```python
from build123d import *

# Parameters (mm, degrees)
F5_R           = 13.25
F5_R_2         = 8
F7_DEPTH       = 50
F4_R           = 13.25
F4_R_2         = 8
F8_DEPTH       = 50
F6_R           = 13.25
F6_R_2         = 8
F9_DEPTH       = 50
F10_DEPTH      = 25
F11_R          = 29
F12_DEPTH      = 3.5
F12_DEPTH_BACK = 2
F13_R          = 3.5
F14_DEPTH      = 51.7280401213
F14_DEPTH_BACK = 25
F17_DEPTH      = 20
F18_R          = 3.5
F19_DEPTH      = 12.9
F20_DEPTH      = 25
F22_W          = 110.3683225811
F22_H          = 78.3186629415
F23_DEPTH      = 25


with BuildPart() as f7:
    # F5 (on line) → F7 (new body)
    with BuildSketch(Plane(origin=(0.8701905284, -0.5024047358, 3.75), x_dir=(0.9745560663, 0.0297636554, -0.2221589485), z_dir=(-0.224143868, 0.1294095226, -0.9659258263))):
        with Locations((12.4405659735, 7.4533997104)):
            Circle(F5_R)
        with Locations((12.4405659735, 7.4533997104)):
            Circle(F5_R_2, mode=Mode.SUBTRACT)
    extrude(amount=-F7_DEPTH)


with BuildPart() as f8:
    # F4 (on line) → F8 (new body)
    with BuildSketch(Plane(origin=(-0.8701905284, -0.5024047358, 3.75), x_dir=(0.9745560663, -0.0297636554, 0.2221589485), z_dir=(0.224143868, 0.1294095226, -0.9659258263))):
        with Locations((-12.544631958, 7.3663704097)):
            Circle(F4_R)
        with Locations((-12.544631958, 7.3663704097)):
            Circle(F4_R_2, mode=Mode.SUBTRACT)
    extrude(amount=-F8_DEPTH)


with BuildPart() as f9:
    # F6 (on line) → F9 (new body)
    with BuildSketch(Plane(origin=(0, 1.0048094716, 3.75), x_dir=(1, 0, 0), z_dir=(0, -0.2588190451, -0.9659258263))):
        with Locations((0, -14.4834918901)):
            Circle(F6_R)
        with Locations((0, -14.4834918901)):
            Circle(F6_R_2, mode=Mode.SUBTRACT)
    extrude(amount=-F9_DEPTH)


with BuildPart() as f10:
    # F0 (on Top) → F10 (new body)
    with BuildSketch(Plane.XY):
        with BuildLine():
            Line((0, 0), (6.0621778265, -3.5))
            ThreePointArc((6.0621778265, -3.5), (9.8988818392, -0.1214749043), (14.998015474, 0.2439914803))
            ThreePointArc((14.998015474, 0.2439914803), (12.9903810568, 7.5), (7.7103105572, 12.8666666667))
            ThreePointArc((7.7103105572, 12.8666666667), (4.8442405666, 8.633420594), (0, 7))
            Line((0, 7), (0, 0))
        make_face()
        with BuildLine():
            Line((-6.0621778265, -3.5), (0, 0))
            Line((0, 0), (0, 7))
            ThreePointArc((0, 7), (-4.8442405666, 8.633420594), (-7.7103105572, 12.8666666667))
            ThreePointArc((-7.7103105572, 12.8666666667), (-12.9903810568, 7.5), (-14.998015474, 0.2439914803))
            ThreePointArc((-14.998015474, 0.2439914803), (-9.8988818392, -0.1214749043), (-6.0621778265, -3.5))
        make_face()
        with BuildLine():
            ThreePointArc((-7.2877049167, -13.110658147), (0, -15), (7.2877049167, -13.110658147))
            ThreePointArc((7.2877049167, -13.110658147), (5.0546412727, -8.5119456897), (6.0621778265, -3.5))
            Line((6.0621778265, -3.5), (0, 0))
            Line((0, 0), (-6.0621778265, -3.5))
            ThreePointArc((-6.0621778265, -3.5), (-5.2629744465, -5.4294476392), (-4.9903810568, -7.5))
            ThreePointArc((-4.9903810568, -7.5), (-5.5869558657, -10.5313850696), (-7.2877049167, -13.110658147))
        make_face()
    extrude(amount=F10_DEPTH)


with BuildPart() as f12:
    # F11 (on Top) → F12 (new body, two sides)
    with BuildSketch(Plane.XY) as f12_sk:
        Circle(F11_R)
    extrude(amount=-F12_DEPTH)
    extrude(f12_sk.sketch, amount=F12_DEPTH_BACK)


with BuildPart() as f14_tool:
    # F13 (on Top) → F14 (new body, two sides)
    with BuildSketch(Plane.XY) as f14_sk:
        Circle(F13_R)
    extrude(amount=F14_DEPTH)
    extrude(f14_sk.sketch, amount=-F14_DEPTH_BACK)


with BuildPart() as f7_1:
    add(f7.part)

    # F14: cut by f14_tool
    add(f14_tool.part, mode=Mode.SUBTRACT)


with BuildPart() as f8_1:
    add(f8.part)

    # F14: cut by f14_tool
    add(f14_tool.part, mode=Mode.SUBTRACT)


with BuildPart() as f9_1:
    add(f9.part)

    # F14: cut by f14_tool
    add(f14_tool.part, mode=Mode.SUBTRACT)


with BuildPart() as f10_1:
    add(f10.part)

    # F14: cut by f14_tool
    add(f14_tool.part, mode=Mode.SUBTRACT)


with BuildPart() as f12_1:
    add(f12.part)

    # F14: cut by f14_tool
    add(f14_tool.part, mode=Mode.SUBTRACT)


with BuildPart() as f7_2:
    add(f7_1.part)

    # F15: union F8, F9, F10, F12
    add(f8_1.part)
    add(f9_1.part)
    add(f10_1.part)
    add(f12_1.part)

    # F16 (on face) → F17 (cut)
    with BuildSketch(Plane(origin=(0, 0, -3.5), x_dir=(1, 0, 0), z_dir=(0, 0, -1))):
        Polygon((-3.275, -5.6724663948), (3.275, -5.6724663948), (6.55, 0), (3.275, 5.6724663948), (-3.275, 5.6724663948), (-6.55, 0), align=None)
    extrude(amount=-F17_DEPTH, mode=Mode.SUBTRACT)

    # F18 (on face) → F19 (join)
    with BuildSketch(Plane.XY.offset(25)):
        with BuildLine():
            ThreePointArc((9.2145774198, 11.8360281756), (0, 7.9883032381), (-9.2145774198, 11.8360281756))
            ThreePointArc((-9.2145774198, 11.8360281756), (-13.0401831697, 7.5480168017), (-14.8529870725, 2.0949403392))
            ThreePointArc((-14.8529870725, 2.0949403392), (-6.9961529284, -3.9893730543), (-5.7610544028, -13.849557833))
            ThreePointArc((-5.7610544028, -13.849557833), (-0.06216489, -14.9998711837), (5.646063326, -13.8968330536))
            ThreePointArc((5.646063326, -13.8968330536), (6.9321877833, -4.0088841204), (14.8609587483, 2.0376224091))
            ThreePointArc((14.8609587483, 2.0376224091), (12.9965398986, 7.4893224435), (9.2145774198, 11.8360281756))
        make_face()
        Circle(F18_R, mode=Mode.SUBTRACT)
    extrude(amount=-F19_DEPTH)

    # F20 (cut): faces of the model
    f20_faces = [f7_2.faces().sort_by_distance(p)[0] for p in [
        (-0.065182715, -22.8612906219, 2),
        (19.8111281547, 11.4386598585, 2),
        (-19.780330483, 11.5571321241, 2),
    ]]
    extrude(f20_faces, amount=-F20_DEPTH, mode=Mode.SUBTRACT)

    # F22 (on offset) → F23 (cut)
    with BuildSketch(Plane.XY.offset(40)):
        with Locations((0.9703096002, 2.6732347906)):
            Rectangle(F22_W, F22_H)
    extrude(amount=F23_DEPTH, mode=Mode.SUBTRACT)


solid = f7_2.part
```
Geometry check sheet. Reference: the model listing, model coordinates, mm. A direction names the side the tool comes from. Give positions to 0.01 mm unless a question says otherwise; leave off trailing zeros.
1. Release check for a two-part mould opening along X. For faces 5 (the face through (25.08, -14.56, -0.79)), 6 (the face through (-12.95, 7.57, 5.92)), 7 (the face through (28, -7, 40)), 8 (the face through (-13.73, -17.03, 20.85)) record: pulls with the +X half, pulls with the -X half, needs draft (parallel to the pull), parting line crosses it, or undercut.
2. Section check A-A, the plane z = 31. Give the number of separate pieces and of enclosed holes in the cut face, and give its area (3 significant figures).
3. Gauge pin test, flat ends, axial feed: pin 1 Ø6 at (y, z) = (-4, 17.5) entering from +X; pin 2 Ø3.5 at (x, y) = (3, 0) entering from -Z; pin 3 Ø4 at (y, z) = (22.5, 35) entering from -X; pin 4 Ø18 at (x, y) = (-17, -9.5) entering from +Z. Record the tip position at first contact, or that the pin passes through.
4. Access from +Z, -Z, +X, -X, +Y, -Y to the whole of each face (thin tool, end or side, straight path). Record for faces 1 (the face through (13, -8, 2)), 2 (the face through (-25.24, -14.28, -1.4)), 3 (the face through (-4, 2, 25)), 4 (the face through (2.8, -2.4, 12.1)).
5. Thickness scan on L1, parallel to Y at x = 3, z = 12; L2, parallel to Y at x = -3, z = 23; L3, parallel to X at y = -18.5, z = 33. Record the ranges inside material, lowest first.
Values follow:
1. face 5: pulls with the +X half
1. face 6: pulls with the -X half
1. face 7: needs draft
1. face 8: undercut
2. separate pieces: 3
2. enclosed holes: 3
2. area: 1,090 mm2
3. pin 1: stops at x = 30.43
3. pin 2: stops at z = 12.1
3. pin 3: stops at x = -13.25
3. pin 4: stops at z = 40
4. face 1: none
4. face 2: -Z, -X, -Y
4. face 3: +Z
4. face 4: -Z
5. L1: y = -14.7 to -5.67, 5.67 to 10.53, 25.89 to 31.57
5. L2: y = -14.7 to -1.8, 1.8 to 13.48, 28.84 to 34.52
5. L3: x = -32.76 to -25.62, -16.3 to -9.16, 9.01 to 16.07, 25.64 to 32.7
